The model under review builds one solid part; all positions refer to its coordinate system, in mm. A direction names the side the tool comes from. Round coordinates to 2 decimals unless told otherwise and drop trailing zeros. Order: outer loops, then holes, each group sorted by start corner. A loop starts at its lowest first (then second) coordinate and runs counter-clockwise, first axis right, second up. Notation, with made-up numbers: M 31.5,75 L 76.5,75 A22 ccw 76.5,94 Z; hole C 5.5,41.25 d10. An arc over 180 degrees is marked long. Answer as a JSON object with one key per item and string values. Group by question number.
1) The part is to be moulded in two halves that separate along Z. For faces 6 (the flat face through (20, 7, -16.75)), 7 (the flat face through (25.75, 7, -18)), 8 (the flat face through (0, 7, 12.7)), say which applies: +Z half, -Z half, draft (parallel to the pull), parting line (faces both ways), or undercut.
2) Consider section C-C, the plane y = 10.25. Write out the cut boundary in (x, z).
3) Insertion check: pin 1 Ø4 at (x, y) = (-22.75, 7) entering from +Z; pin 2 Ø1 at (y, z) = (6.5, -10.5) entering from +X; pin 3 Ø2 at (y, z) = (6, -13.75) entering from +X. Each pin has a flat end and moves straight along its axis. Give the tip position at first contact, or say it passes through.
4) To check wall thickness, follow line 1 (Z direction, x = -0.5, y = 5.75); line 2 (X direction, y = 6.25, z = 8); line 3 (Z direction, x = 11.5, y = 6). State the ranges of each line that lie inside material, in increasing order.
5) For faces 1 (the flat face through (0, 7, -18.75)), 2 (the cylindrical face through (-13, 6, -15)), 3 (the cylindrical face through (13, 6, 15)), 4 (the flat face through (-12.7, 7, 0)), 5 (the flat face through (-25.75, 7, -18)), list the 3-axis set-ups (+Z, -Z, +X, -X, +Y, -Y) from which the entire face can be reached by the end or side of a thin tool; tool diameter is ignored.
6) Consider section D-D, the plane y = 8. Write out the cut boundary in (x, z).
7) Consider section B-B, the plane z = -3. Write out the cut boundary in (x, y).
8) Consider section A-A, the plane x = -1. Write out the cut boundary in (y, z), then the cut area to 3 significant figures.
```python
from build123d import *

# Parameters (mm, degrees)
SKETCH1_W                      = 33.5
SKETCH1_H                      = 33.5
BOSS_EXTRUDE1_DEPTH            = 70
M3X0_5_TAPPED_HOLE1_D          = 2.5
M3X0_5_TAPPED_HOLE1_DEPTH      = 7.62
M3X0_5_TAPPED_HOLE1_TIP        = 0.751075774
M3X0_5_TAPPED_HOLE2_D          = 2.5
M3X0_5_TAPPED_HOLE2_DEPTH      = 7.62
M3X0_5_TAPPED_HOLE2_TIP        = 0.751075774
SKETCH7_W                      = 6
SKETCH7_H                      = 50
BOSS_EXTRUDE2_DEPTH            = 3
SKETCH8_W                      = 6
SKETCH8_H                      = 50
BOSS_EXTRUDE3_DEPTH            = 3
SKETCH10_W                     = 1.7
SKETCH10_H                     = 33.5
M3_CLEARANCE_HOLE1_AT_2_COUNT  = 2
M3_CLEARANCE_HOLE1_AT_2_PITCH  = 25
M3_CLEARANCE_HOLE1_AT_3_COUNT  = 2
M3_CLEARANCE_HOLE1_AT_3_PITCH  = 39.5
M3_CLEARANCE_HOLE1_AT_4_COUNT  = 2
M3_CLEARANCE_HOLE1_AT_4_PITCH  = 46.746657635
SKETCH12_W                     = 33.5
SKETCH12_H                     = 45
CUT_EXTRUDE2_DEPTH             = 32.5
M3X0_5_TAPPED_HOLE3_AT_2_COUNT = 2
M3X0_5_TAPPED_HOLE3_AT_2_PITCH = 27.5
SKETCH16_W                     = 45.5
SKETCH16_H                     = 59.85996371
CUT_EXTRUDE3_DEPTH             = 34.5
SKETCH17_W                     = 51.5
SKETCH17_H                     = 11
BOSS_EXTRUDE4_DEPTH            = 2
SKETCH22_W                     = 51.5
SKETCH22_H                     = 3.322905466
CUT_EXTRUDE5_DEPTH             = 36.5
M3_CLEARANCE_HOLE3_D           = 3.4
SKETCH24_W                     = 25.4
SKETCH24_H                     = 25.4
CUT_EXTRUDE6_DEPTH             = 8.677094534


with BuildPart() as part:
    # Sketch1 → Boss-Extrude1 (new body)
    with BuildSketch(Plane(origin=(0, 0, 0), x_dir=(1, 0, 0), z_dir=(0, 1, 0))):
        Rectangle(SKETCH1_W, SKETCH1_H)
    extrude(amount=BOSS_EXTRUDE1_DEPTH)

    # M3x0.5 Tapped Hole1
    with Locations(Plane(origin=(13.75, 70, 13.75), x_dir=(0, 0, 1), z_dir=(0, 1, 0))):
        with Locations((0, 0), (-27.5, -27.5)):
            Hole(M3X0_5_TAPPED_HOLE1_D / 2, depth=M3X0_5_TAPPED_HOLE1_DEPTH)
            with Locations((0, 0, -(M3X0_5_TAPPED_HOLE1_DEPTH + M3X0_5_TAPPED_HOLE1_TIP / 2))):  # 118° drill point
                Cone(0, M3X0_5_TAPPED_HOLE1_D / 2, M3X0_5_TAPPED_HOLE1_TIP, mode=Mode.SUBTRACT)

    # M3x0.5 Tapped Hole2
    with Locations(Plane(origin=(16.75, 6, 13.75), x_dir=(0, 0, 1), z_dir=(1, 0, 0))):
        with Locations((0, 0), (-27.5, 0)):
            Hole(M3X0_5_TAPPED_HOLE2_D / 2, depth=M3X0_5_TAPPED_HOLE2_DEPTH)
            with Locations((0, 0, -(M3X0_5_TAPPED_HOLE2_DEPTH + M3X0_5_TAPPED_HOLE2_TIP / 2))):  # 118° drill point
                Cone(0, M3X0_5_TAPPED_HOLE2_D / 2, M3X0_5_TAPPED_HOLE2_TIP, mode=Mode.SUBTRACT)

    # Sketch12 → Cut-Extrude2 (cut)
    with BuildSketch(Plane.XY.offset(16.75)):
        with Locations((0, 35.5)):
            Rectangle(SKETCH12_W, SKETCH12_H)
    extrude(amount=-CUT_EXTRUDE2_DEPTH, mode=Mode.SUBTRACT)

    # Sketch13 → M3x0.5 Tapped Hole3 (revolve, cut)
    with BuildSketch(Plane(origin=(-16.75, 6, -13.75), x_dir=(0, 0, 1), z_dir=(0, 1, 0))):
        Polygon((0, 0), (0, 8.371075774), (1.25, 7.62), (1.25, 0), align=None)
    m3x0_5_tapped_hole3 = revolve(axis=Axis((-23.1, 6, -13.75), (1, 0, 0)), mode=Mode.SUBTRACT)

    # M3x0.5 Tapped Hole3 at 2: M3x0.5 Tapped Hole3 ×2
    with Locations(*[(0, 0, i * M3X0_5_TAPPED_HOLE3_AT_2_PITCH) for i in range(1, M3X0_5_TAPPED_HOLE3_AT_2_COUNT)]):
        add(m3x0_5_tapped_hole3, mode=Mode.SUBTRACT)


with BuildPart() as body_2:
    # Sketch7 → Boss-Extrude2 (new body)
    with BuildSketch(Plane(origin=(0, 0, -16.75), x_dir=(-1, 0, 0), z_dir=(0, 0, -1))):
        with Locations((-19.75, 36)):
            Rectangle(SKETCH7_W, SKETCH7_H)
    extrude(amount=-BOSS_EXTRUDE2_DEPTH)

    # Sketch10 → M3 Clearance Hole1 (revolve, cut)
    with BuildSketch(Plane(origin=(19.75, 51, -16.75), x_dir=(0, 1, 0), z_dir=(1, 0, 0))):
        with Locations((0.85, 16.75)):
            Rectangle(SKETCH10_W, SKETCH10_H)
    m3_clearance_hole1 = revolve(axis=Axis((19.75, 51, -23.1), (0, 0, 1)), mode=Mode.SUBTRACT)

    # M3 Clearance Hole1 at 2: M3 Clearance Hole1 ×2
    with Locations(*[(0, -i * M3_CLEARANCE_HOLE1_AT_2_PITCH, 0) for i in range(1, M3_CLEARANCE_HOLE1_AT_2_COUNT)]):
        add(m3_clearance_hole1, mode=Mode.SUBTRACT)


with BuildPart() as body_3:
    # Sketch8 → Boss-Extrude3 (new body)
    with BuildSketch(Plane(origin=(0, 0, -16.75), x_dir=(-1, 0, 0), z_dir=(0, 0, -1))):
        with Locations((19.75, 36)):
            Rectangle(SKETCH8_W, SKETCH8_H)
    extrude(amount=-BOSS_EXTRUDE3_DEPTH)

    # M3 Clearance Hole1 at 3: M3 Clearance Hole1 ×2
    with Locations(*[(-i * M3_CLEARANCE_HOLE1_AT_3_PITCH, 0, 0) for i in range(1, M3_CLEARANCE_HOLE1_AT_3_COUNT)]):
        add(m3_clearance_hole1, mode=Mode.SUBTRACT)

    # M3 Clearance Hole1 at 4: M3 Clearance Hole1 ×2
    with Locations(*[Vector(-0.844980197, -0.534797593, 0) * (i * M3_CLEARANCE_HOLE1_AT_4_PITCH) for i in range(1, M3_CLEARANCE_HOLE1_AT_4_COUNT)]):
        add(m3_clearance_hole1, mode=Mode.SUBTRACT)


with BuildPart() as cut_extrude3_tool:
    # Sketch16 → Cut-Extrude3 (new body, through all)
    with BuildSketch(Plane.XY.offset(16.75)):
        with Locations((0, 40.929981855)):
            Rectangle(SKETCH16_W, SKETCH16_H)
    extrude(amount=-CUT_EXTRUDE3_DEPTH)


with BuildPart() as part_1:
    add(part.part)

    # Cut-Extrude3: cut by cut_extrude3_tool
    add(cut_extrude3_tool.part, mode=Mode.SUBTRACT)

    # Sketch17 → Boss-Extrude4 (add)
    with BuildSketch(Plane(origin=(0, 0, -16.75), x_dir=(-1, 0, 0), z_dir=(0, 0, -1))):
        with Locations((0, 5.5)):
            Rectangle(SKETCH17_W, SKETCH17_H)
    extrude(amount=BOSS_EXTRUDE4_DEPTH)

    # Sketch22 → Cut-Extrude5 (cut, through all)
    with BuildSketch(Plane(origin=(0, 0, -18.75), x_dir=(-1, 0, 0), z_dir=(0, 0, -1))):
        with Locations((0, 1.661452733)):
            Rectangle(SKETCH22_W, SKETCH22_H)
    extrude(amount=-CUT_EXTRUDE5_DEPTH, mode=Mode.SUBTRACT)

    # M3 Clearance Hole3 (through all)
    with Locations(Plane(origin=(22.75, 7, -16.75), x_dir=(1, 0, 0), z_dir=(0, 0, 1))):
        with Locations((0, 0), (-45.5, 0)):
            Hole(M3_CLEARANCE_HOLE3_D / 2)

    # Sketch24 → Cut-Extrude6 (cut, through all)
    with BuildSketch(Plane(origin=(0, 11, 0), x_dir=(1, 0, 0), z_dir=(0, 1, 0))):
        Rectangle(SKETCH24_W, SKETCH24_H)
    extrude(amount=-CUT_EXTRUDE6_DEPTH, mode=Mode.SUBTRACT)


with BuildPart() as body_2_1:
    add(body_2.part)

    # Cut-Extrude3: cut by cut_extrude3_tool
    add(cut_extrude3_tool.part, mode=Mode.SUBTRACT)


with BuildPart() as body_3_1:
    add(body_3.part)

    # Cut-Extrude3: cut by cut_extrude3_tool
    add(cut_extrude3_tool.part, mode=Mode.SUBTRACT)


solid = part_1.part
```
Results list:
{
 "1": {"face 6": "+Z half", "face 7": "draft", "face 8": "undercut"},
 "2": {"outline": "M -25.75,-18.75 L 25.75,-18.75 L 25.75,-16.75 L 16.75,-16.75 L 16.75,16.75 L -16.75,16.75 L -16.75,-16.75 L -25.75,-16.75 Z; hole M -12.7,-12.7 L 12.7,-12.7 L 12.7,12.7 L -12.7,12.7 Z"},
 "3": {"pin 1": "z = -16.75", "pin 2": "x = 16.75", "pin 3": "x = 8.98"},
 "4": {"line 1": "-18.75 to -12.7, 12.7 to 16.75", "line 2": "-16.75 to -12.7, 12.7 to 16.75", "line 3": "-18.75 to -15, 15 to 16.75"},
 "5": {"face 1": "-Z, +X, -X, +Y, -Y", "face 2": "-X", "face 3": "+X", "face 4": "+Y, -Y", "face 5": "+Z, -Z, -X, +Y, -Y"},
 "6": {"outline": "M -25.75,-18.75 L -24.12,-18.75 L -24.12,-16.75 L -25.75,-16.75 Z; M -21.38,-18.75 L 21.38,-18.75 L 21.38,-16.75 L 16.75,-16.75 L 16.75,16.75 L -16.75,16.75 L -16.75,-16.75 L -21.38,-16.75 Z; M 24.12,-18.75 L 25.75,-18.75 L 25.75,-16.75 L 24.12,-16.75 Z; hole M -12.7,-12.7 L 12.7,-12.7 L 12.7,12.7 L -12.7,12.7 Z"},
 "7": {"outline": "M -16.75,3.32 L -12.7,3.32 L -12.7,11 L -16.75,11 Z; M 12.7,3.32 L 16.75,3.32 L 16.75,11 L 12.7,11 Z"},
 "8": {"outline": "M 3.32,-18.75 L 11,-18.75 L 11,-12.7 L 3.32,-12.7 Z; M 3.32,12.7 L 11,12.7 L 11,16.75 L 3.32,16.75 Z", "area": "77.5 mm^2"}
}
